Could you check a few things on this model? Use its own coordinates, in mm. Face numbers are marked on the shaded views. Coordinates: 2 decimals unless noted, no trailing zeros. Loops run counter-clockwise (first coordinate to the right, second up) from the corner with the lowest first, then second, coordinate; pieces in that order, holes last. Notation, with made-up numbers: M 75.5,50.5 L 115.5,50.5 A25 ccw 115.5,68.5 Z; hole C 61.25,-13.5 d3. An arc over 180 degrees is marked long. Use one line per item in the form item = value. Start each with the question number.
Autodesk Inventor part; units mm, degrees
ref_plane "YZ Plane" through (0, 0, 0) normal (1, 0, 0) x (0, 1, 0)
ref_plane "XZ Plane" through (0, 0, 0) normal (0, 1, 0) x (-1, 0, 0)
ref_plane "XY Plane" through (0, 0, 0) normal (0, 0, 1) x (1, 0, 0)
sketch "Sketch1" plane through (0, 0, 0) normal (0, 0, 1) x (1, 0, 0)
  line L0 (-139.7, 31.75) -> (139.7, 31.75)
  line L1 (139.7, 31.75) -> (139.7, -31.75)
  line L2 (139.7, -31.75) -> (-139.7, -31.75)
  line L3 (-139.7, -31.75) -> (-139.7, 31.75)
  point P0 (0, 0)
  point P1 (0, 31.75)
  point P2 (139.7, 0)
  dimension "d0" = 279.4
  dimension "d1" = 63.5
extrude "Extrusion1" add sketch "Sketch1" along normal blind 43.18
sketch "Sketch2" plane through (0, 0, 43.18) normal (0, 0, 1) x (1, 0, 0)
  line L0 (-139.7, -31.75) -> (139.7, -31.75)
  line L1 (-138.1125, 30.1625) -> (138.1125, 30.1625)
  line L2 (138.1125, 30.1625) -> (138.1125, -31.75)
  line L3 (138.1125, -31.75) -> (-138.1125, -31.75)
  line L4 (-138.1125, -31.75) -> (-138.1125, 30.1625)
  line L5 (139.7, -31.75) -> (139.7, 31.75)
  line L6 (139.7, 31.75) -> (-139.7, 31.75)
  line L7 (-139.7, 31.75) -> (-139.7, -31.75)
  point P0 (0, 0)
  point P1 (-138.1125, -31.75)
  dimension "d4" = 1.5875
  dimension "d5" = 1.5875
  dimension "d6" = 1.5875
extrude "Extrusion2" cut sketch "Sketch2" against normal up to surface (43.18 mm away) contours L4 L1 L2 L0
sketch "Sketch3" plane through (-138.1125, -31.75, 43.18) normal (1, 0, 0) x (0, 0, -1)
  circle A0 centre (21.59, 41.5925) radius 5.05
  line L0 (0, 61.9125) -> (43.18, 61.9125)
  circle A1 centre (21.59, 21.2725) radius 1.5875
  line L1 (43.18, 63.5) -> (0, 63.5)
  point P0 (43.18, 31.75)
  point P1 (21.59, 63.5)
  dimension "d9" = 10.1
  dimension "d10" = 20.32
  dimension "d13" = 3.175
  dimension "d15" = 20.32
extrude "Extrusion3" cut sketch "Sketch3" along normal through all both and the other way through all
sketch "Sketch4" plane through (139.7, -31.75, 0) normal (1, 0, 0) x (0, 0, -1)
  circle A0 centre (-12.7, 26.3525) radius 2.3813
  line L0 (0, 63.5) -> (-43.18, 63.5) construction
  line L1 (-21.59, 63.5) -> (-21.59, -3.1611) construction
  line L2 (0, 0) -> (0, 63.5)
  circle A1 centre (-21.59, 41.5925) radius 5.05
  circle A2 centre (-30.48, 26.3525) radius 2.3813
  point P0 (0, 31.75)
  dimension "d16" = 12.7
  dimension "d17" = 15.24
  dimension "d18" = 4.7625
extrude "Extrusion4" cut sketch "Sketch4" against normal up to surface (1.5875 mm away) contours A0 | A2
sketch "Sketch5" plane through (-139.7, -31.75, 0) normal (-1, 0, 0) x (0, 0, 1)
  circle A0 centre (21.59, 41.5925) radius 5.05 construction
  line L0 (21.59, 41.5925) -> (21.59, 66.4825) construction
  line L1 (21.59, 41.5925) -> (51.2225, 41.5925) construction
  circle A1 centre (37.09, 57.0925) radius 1.5875
  circle A2 centre (6.09, 57.0925) radius 1.5875
  circle A3 centre (37.09, 26.0925) radius 1.5875
  circle A4 centre (6.09, 26.0925) radius 1.5875
  point P0 (0, 31.75)
  dimension "d21" = 3.175
  dimension "d22" = 15.5
  dimension "d23" = 15.5
extrude "Extrusion5" cut sketch "Sketch5" against normal up to surface (1.5875 mm away)
sketch "Sketch6" plane through (0, 0, 43.18) normal (0, 0, 1) x (1, 0, 0)
  line L0 (138.1125, 30.1625) -> (138.1125, -31.75)
  line L1 (138.1125, 30.1625) -> (147.9517, 30.1625)
  line L2 (147.9517, 30.1625) -> (147.9517, 39.5232)
  line L3 (147.9517, 39.5232) -> (138.1125, 39.5232)
  line L4 (138.1125, 39.5232) -> (138.1125, 30.1625)
  line L5 (138.1125, 30.1625) -> (-192.5476, 30.1625)
  line L6 (-192.5476, 30.1625) -> (-192.5476, 49.9994)
  line L7 (-192.5476, 49.9994) -> (138.1125, 49.9994)
  line L8 (138.1125, 49.9994) -> (138.1125, 30.1625)
  line L9 (-192.5476, 30.1625) -> (-74.3706, 30.1625)
  line L10 (-74.3706, 30.1625) -> (-74.3706, -79.1708)
  line L11 (-74.3706, -79.1708) -> (-192.5476, -79.1708)
  line L12 (-192.5476, -79.1708) -> (-192.5476, 30.1625)
  point P0 (0, 0)
extrude "Extrusion6" cut sketch "Sketch6" against normal through all
sketch "Sketch7" plane through (139.7, -31.75, 43.18) normal (1, 0, 0) x (0, 0, -1)
  line L0 (43.18, 61.9125) -> (0, 61.9125)
  line L1 (0, 0) -> (0, 61.9125)
  line L2 (43.18, 0) -> (0, 0)
  line L3 (43.18, 0) -> (43.18, 61.9125)
  circle A0 centre (21.59, 21.2725) radius 1.5875
  circle A1 centre (21.59, 41.5925) radius 5.05
  circle A2 centre (30.48, 26.3525) radius 2.3813
  circle A3 centre (12.7, 26.3525) radius 2.3813
  point P0 (43.18, 31.75)
extrude "Extrusion7" add sketch "Sketch7" against normal blind 6.35
sketch "Sketch8" plane through (139.7, 30.1625, 43.18) normal (0, 1, 0) x (1, 0, 0)
  line L0 (-6.35, 0) -> (0, 0)
  line L1 (-6.35, 0) -> (0, 0)
  line L2 (-3.175, 0) -> (-3.175, 6.35)
  line L3 (-6.35, 43.18) -> (0, 43.18)
  line L4 (-3.175, 43.18) -> (-3.175, 36.83)
  point P0 (-139.7, 43.18)
  dimension "d30" = 6.35
  dimension "d31" = 6.35
hole "Hole1" at (136.525, 30.1625, 36.83) at (136.525, 30.1625, 6.35) direction (0, -1, 0) diameter 3.6576 depth 22.479 tip angle 118
properties part number "Bracket(right)"
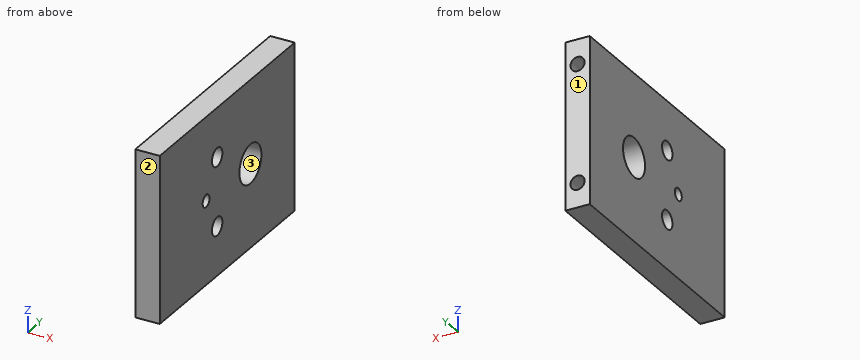
Item 1: I want a section at C-C (z = 12.7). Write out the boundary of the cut face in (x, y), plus the area to 3 significant figures.
Item 2: I want a section at B-B (y = 14). Write out the boundary of the cut face in (x, z) (3 decimals).
Item 3: Please list where these lines run through material, in increasing order: line 1 along Z through (x, y) = (136.5, 20); line 2 along X through (y, z) = (18.25, 6.35); line 3 along Z through (x, y) = (135.5, 23).
Item 4: I want a section at D-D (y = 21). Write out the boundary of the cut face in (x, z) (3 decimals), plus the area to 3 significant figures.
Item 5: I'm going to push flat-ended pins straight in: P1, Ø3, axis at x = 136.525, z = 36.83, coming from the +Y side; P2, Ø2, axis at x = 136.525, z = 6.35, coming from the +Y side. Where does each tip first touch, or does it pass through?
Item 6: I want a section at A-A (z = 21.59). Count the separate pieces of the cut face and the enclosed holes in it, plus the area to 3 significant figures.
Item 7: Thinking about a two-plate mould opening in Y: for the marked faces 1, 2 and 3, which applies, pulls with the +Y half, pulls with the -Y half, needs draft (parallel to the pull), parting line crosses it, or undercut?
Worked answers:
q1.outline = M 133.35,-31.75 L 139.7,-31.75 L 139.7,-7.78 L 133.35,-7.78 Z; M 133.35,-3.02 L 139.7,-3.02 L 139.7,30.16 L 133.35,30.16 Z
q1.area = 363 mm²
q2.outline = M 133.35,0 L 139.7,0 L 139.7,18.723 L 133.35,18.723 Z; M 133.35,24.457 L 139.7,24.457 L 139.7,43.18 L 133.35,43.18 Z; hole C 136.525,6.35 d3.658; hole C 136.525,36.83 d3.658
q3.line_1 = 0 to 4.52, 8.18 to 35, 38.66 to 43.18
q3.line_2 = 133.35 to 134.7, 138.35 to 139.7
q3.line_3 = 0 to 4.84, 7.86 to 35.32, 38.34 to 43.18
q4.outline = M 133.35,0 L 139.7,0 L 139.7,43.18 L 133.35,43.18 Z; hole C 136.525,6.35 d3.658; hole C 136.525,36.83 d3.658
q4.area = 253 mm²
q5.P1 = 7.49
q5.P2 = 7.19
q6.separate_pieces = 3
q6.enclosed_holes = 0
q6.area = 309 mm²
q7.face_1 = pulls with the +Y half
q7.face_2 = pulls with the -Y half
q7.face_3 = undercut
